from build123d import *


with BuildPart() as part:
    # Sketch1 → Revolve1 (revolve)
    with BuildSketch(Plane.XY, mode=Mode.PRIVATE) as revolve1_sk:
        with BuildLine():
            ThreePointArc((-6.35, 63.5), (0, 79.375), (6.35, 63.5))
            Line((6.35, 63.5), (6.35, 50.8))
            Line((6.35, 50.8), (3.175, 50.8))
            Line((3.175, 50.8), (3.175, 44.45))
            Line((3.175, 44.45), (-3.175, 44.45))
            Line((-3.175, 44.45), (-3.175, 50.8))
            Line((-3.175, 50.8), (-6.35, 50.8))
            Line((-6.35, 50.8), (-6.35, 63.5))
        make_face()
    revolve(revolve1_sk.sketch.rotate(Axis((0, 0, 0), (1, 0, 0)), 90), axis=Axis((0, 0, 0), (1, 0, 0)))


solid = part.part
The model under review builds one solid part; all positions refer to its coordinate system, in mm. A direction names the side the tool comes from. Give positions to 0.01 mm unless a question says otherwise; leave off trailing zeros. Write each loop counter-clockwise with the first axis right and the second up, starting at its lowest first coordinate (ties: lowest second). Pieces come first, ordered by that corner, then holes. Notation, with made-up numbers: M 27.5,2.25 L 76.5,2.25 A16 ccw 76.5,18.25 Z; hole C 66,3 d8. An arc over 180 degrees is marked long. One line per question, with ' | ' between items. Start each with the question number.
Item 1: For pin 1 (10 mm diameter, centred on y = 48, z = -21, fed in from -X); pin 2 (12 mm diameter, centred on y = 57, z = -23.5, fed in from -X); pin 3 (5 mm diameter, centred on y = 48.5, z = 31, fed in from +X), all flat-tipped, find the tip position at first contact; note any pin that passes through.
Item 2: We need section C-C on x = 1.25. Write out the cut boundary in (y, z).
Item 3: Wall thickness on line 1 (Y direction, x = -0.5, z = 0); line 2 (Y direction, x = 4.9, z = 0); line 3 (Z direction, x = -6.5, y = 15.5): over which ranges is each line inside the solid? List them lowest first. Write a range as from..to.
Item 4: For faces 1 (the cylindrical face through (0, -30, -32.8)), 2 (the cylindrical face through (4.74, 30.911, -40.313)), 3 (the flat face through (-3.175, 45, 0)), list the 3-axis set-ups (+Z, -Z, +X, -X, +Y, -Y) from which the entire face can be reached by the end or side of a thin tool; tool diameter is ignored.
Results found:
1) pin 1: stops at x = -6.35 | pin 2: stops at x = -8.86 | pin 3: stops at x = 6.35
2) outline: C 0,0 d158.58; hole C 0,0 d88.9
3) line 1: y = -79.36..-44.45, 44.45..79.36 | line 2: y = -77.96..-50.8, 50.8..77.96 | line 3: z = -75.11..-61.73, 61.73..75.11
4) face 1: +X, -X | face 2: +X | face 3: -X
